Could you check a few things on this model? Use its own coordinates, in mm. Give positions to 0.01 mm unless a question says otherwise; leave off trailing zeros. Order: outer loops, then holes, each group sorted by start corner. A loop starts at its lowest first (then second) coordinate and runs counter-clockwise, first axis right, second up. Notation, with made-up numbers: (14, 16.5) -> (65, 16.5) arc R13 cw to (65, 33.5) -> close; hole circle Ø6 at (48.5, 24). An arc over 180 degrees is marked (long way). Answer as CSV lines item,"result". Start each with the question number.
(1) I need wall thicknesses on L1, parallel to X at y = 4, z = 2; L2, parallel to X at y = 5, z = 2.5; L3, parallel to X at y = 4, z = 7. Which ranges of each line are inside material? Lowest first, please.
(2) Will this pin go through, and if not, where does the flat tip stop? pin 1 Ø3 at (y, z) = (1.5, 3.5) entering from +X.
(3) We'd pull the mould along X, two halves only. Please class faces 1 (the face through (33, 8, 5)), 2 (the face through (0, 4, 7)), 3 (the face through (9.259, 4.056, 4.975)): released by +X, released by -X, zero draft, split by the parting line, or undercut.
(4) I want a section at A-A (z = 6). Please give me the cut outline in (x, y).
(5) I want a section at B-B (y = 1.5). Please give me the cut outline in (x, z), plus the area to 3 significant figures.
```python
from build123d import *

# Parameters (mm, degrees)
F1_DEPTH = 10
F2_R     = 5
F3_R     = 4.975574
F4_DEPTH = 25
F5_R     = 1.756999
F6_DEPTH = 25


with BuildPart() as f1:
    # F0 (on Top) → F1 (new body)
    with BuildSketch(Plane.XY):
        with BuildLine():
            Line((0, 8), (0, 0))
            Line((0, 0), (66, 0))
            ThreePointArc((66, 0), (68.828427, 1.171573), (70, 4))
            ThreePointArc((70, 4), (68.828427, 6.828427), (66, 8))
            Line((66, 8), (0, 8))
        make_face()
    extrude(amount=F1_DEPTH)

    # F2
    f2_edges = [f1.edges().sort_by_distance(p)[0] for p in [
        (0, 4, 0),
    ]]
    fillet(f2_edges, radius=F2_R)

    # F3 (on face) → F4 (cut)
    with BuildSketch(Plane(origin=(0, 8, 0), x_dir=(-1, 0, 0), z_dir=(0, 1, 0))):
        with Locations((-9.348009, 0)):
            Circle(F3_R)
    extrude(amount=-F4_DEPTH, mode=Mode.SUBTRACT)

    # F5 (on face) → F6 (cut)
    with BuildSketch(Plane(origin=(0, 0, 0), x_dir=(1, 0, 0), z_dir=(0, 0, -1))):
        with Locations((66.500589, -4)):
            Circle(F5_R)
    extrude(amount=-F6_DEPTH, mode=Mode.SUBTRACT)


solid = f1.part
```
Final values:
1,L1,"1 to 4.79, 13.9 to 64.74, 68.26 to 70"
1,L2,"0.67 to 5.05, 13.65 to 65.06, 67.95 to 69.87"
1,L3,"0 to 64.74, 68.26 to 70"
2,pin 1,"x = 69.87"
3,face 1,"zero draft"
3,face 2,"released by -X"
3,face 3,"undercut"
4,outline,"(0, 0) -> (66, 0) arc R4 ccw to (66, 8) -> (0, 8) -> close; hole circle Ø3.51 at (66.5, 4)"
5,outline,"(0, 5) arc R5 ccw to (4.37, 0.04) arc R4.98 cw to (14.32, 0) -> (69.12, 0) -> (69.12, 10) -> (0, 10) -> close"
5,area,"647 mm²"
